Work out the finished part from the listing and answer in its coordinate system (mm). Face numbers are marked on the shaded views. A direction names the side the tool comes from. Round coordinates to 2 decimals unless told otherwise and drop trailing zeros. Loops run counter-clockwise (first coordinate to the right, second up) from the corner with the lowest first, then second, coordinate; pieces in that order, holes last. Notation, with made-up numbers: (23.25, 18) - (45.25, 18) arc R5 ccw to (45.25, 23) - close; hole circle Ø4 at (-21, -1). An arc over 180 degrees is marked (long way). Return JSON: item names as keys, results as strings.
from build123d import *

# Parameters (mm, degrees)
SKETCH1_R           = 2
SKETCH1_R_2         = 13.2
SKETCH1_R_3         = 11.2
BOSS_EXTRUDE1_DEPTH = 3.6
SKETCH2_R           = 2
SKETCH2_R_2         = 5.25
BOSS_EXTRUDE2_DEPTH = 2
SKETCH3_R           = 2
CUT_EXTRUDE1_DEPTH  = 2
SKETCH4_R           = 1.8
BOSS_EXTRUDE3_DEPTH = 3.6


with BuildPart() as part:
    # Sketch1 → Boss-Extrude1 (new body)
    # profile 1 of 3: a face of its own
    with BuildSketch(Plane(origin=(0, 0, 0), x_dir=(1, 0, 0), z_dir=(0, 1, 0))):
        with BuildLine():
            ThreePointArc((-6.939428571, -11.228727938), (-13.2, 0), (-6.939428571, 11.228727938))
            Line((-6.939428571, 11.228727938), (-19.602857143, 3.40264483))
            ThreePointArc((-19.602857143, 3.40264483), (-21.5, 0), (-19.602857143, -3.40264483))
            Line((-19.602857143, -3.40264483), (-6.939428571, -11.228727938))
        make_face()
        with Locations(Location((-17.5, 0, 0), (0, 0, 270))):
            Circle(SKETCH1_R, mode=Mode.SUBTRACT)
    # profile 2 of 3: a face of its own
    with BuildSketch(Plane(origin=(0, 0, 0), x_dir=(1, 0, 0), z_dir=(0, 1, 0))):
        Circle(SKETCH1_R_2)
        with Locations(Location((0, 0, 0), (0, 0, 270))):
            Circle(SKETCH1_R_3, mode=Mode.SUBTRACT)
    # profile 3 of 3: a face of its own
    with BuildSketch(Plane(origin=(0, 0, 0), x_dir=(1, 0, 0), z_dir=(0, 1, 0))):
        with BuildLine():
            Line((19.602857143, 3.40264483), (6.939428571, 11.228727938))
            ThreePointArc((6.939428571, 11.228727938), (11.529103546, 6.428045693), (13.2, 0))
            ThreePointArc((13.2, 0), (11.529103546, -6.428045693), (6.939428571, -11.228727938))
            Line((6.939428571, -11.228727938), (19.602857143, -3.40264483))
            ThreePointArc((19.602857143, -3.40264483), (21.5, 0), (19.602857143, 3.40264483))
        make_face()
        with Locations(Location((17.5, 0, 0), (0, 0, 270))):
            Circle(SKETCH1_R, mode=Mode.SUBTRACT)
    extrude(amount=BOSS_EXTRUDE1_DEPTH)

    # Sketch2 → Boss-Extrude2 (add)
    with BuildSketch(Plane(origin=(0, 3.6, 0), x_dir=(1, 0, 0), z_dir=(0, 1, 0))):
        with BuildLine():
            Line((-6.939428571, 11.228727938), (-19.602857143, 3.40264483))
            ThreePointArc((-19.602857143, 3.40264483), (-21.5, 0), (-19.602857143, -3.40264483))
            Line((-19.602857143, -3.40264483), (-6.939428571, -11.228727938))
            ThreePointArc((-6.939428571, -11.228727938), (0, -13.2), (6.939428571, -11.228727938))
            Line((6.939428571, -11.228727938), (19.602857143, -3.40264483))
            ThreePointArc((19.602857143, -3.40264483), (21.5, 0), (19.602857143, 3.40264483))
            Line((19.602857143, 3.40264483), (6.939428571, 11.228727938))
            ThreePointArc((6.939428571, 11.228727938), (0, 13.2), (-6.939428571, 11.228727938))
        make_face()
        with Locations(Location((17.5, 0, 0), (0, 0, 270))):
            Circle(SKETCH2_R, mode=Mode.SUBTRACT)
        with Locations(Location((-17.5, 0, 0), (0, 0, 270))):
            Circle(SKETCH2_R, mode=Mode.SUBTRACT)
        with Locations(Location((0, 0, 0), (0, 0, 270))):
            Circle(SKETCH2_R_2, mode=Mode.SUBTRACT)
    extrude(amount=BOSS_EXTRUDE2_DEPTH)

    # Sketch3 → Cut-Extrude1 (cut)
    with BuildSketch(Plane(origin=(0, 5.6, 0), x_dir=(1, 0, 0), z_dir=(0, 1, 0))):
        with Locations(Location((5.727564928, 5.727564928, 0), (0, 0, 270))):
            Circle(SKETCH3_R)
        with Locations(Location((-5.727564928, -5.727564928, 0), (0, 0, 270))):
            Circle(SKETCH3_R)
    extrude(amount=-CUT_EXTRUDE1_DEPTH, mode=Mode.SUBTRACT)

    # Sketch4 → Boss-Extrude3 (add)
    with BuildSketch(Plane.XZ.offset(-3.6)):
        with Locations(Location((5.727564928, 5.727564928, 0), (0, 0, 90))):
            Circle(SKETCH4_R)
        with Locations(Location((-5.727564928, -5.727564928, 0), (0, 0, 90))):
            Circle(SKETCH4_R)
    extrude(amount=BOSS_EXTRUDE3_DEPTH)


solid = part.part
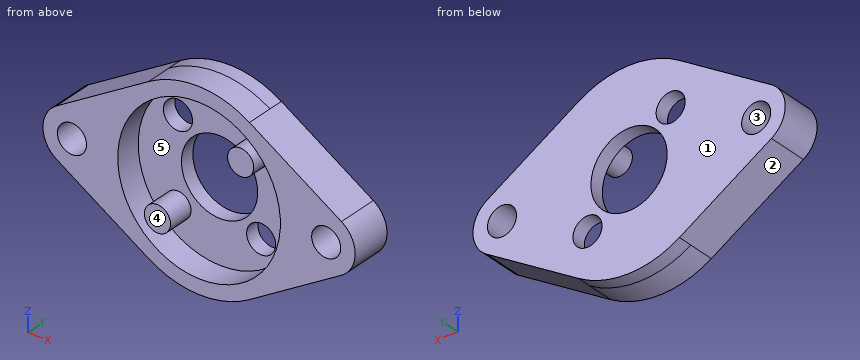
1) Determine the mould class of the marked faces 1, 2 and 3 for opening direction X: pulls with the +X half, pulls with the -X half, needs draft (parallel to the pull), parting line crosses it, or undercut.
Verdict:
{"face 1": "needs draft", "face 2": "pulls with the -X half", "face 3": "undercut"}
2) Flat-ended cylindrical pins translate along their axes: pin 1 (3 mm diameter, centred on x = 0, z = -9, fed in from -Y); pin 2 (2 mm diameter, centred on x = 6, y = 4.5, fed in from +Z); pin 3 (2 mm diameter, centred on x = 12.5, y = 1.5, fed in from -Z). Find the tip coordinate at first contact, or state that the pin passes through.
Verdict:
{"pin 1": "stops at y = 3.6", "pin 2": "stops at z = 12.22", "pin 3": "stops at z = -8.41"}
3) Section C-C (x = 17.5) is taken. Give the vertices of the cut face in (y, z).
Verdict:
{"outline": "(0, -4.7) - (5.6, -4.7) - (5.6, -2) - (0, -2) - close; (0, 2) - (5.6, 2) - (5.6, 4.7) - (0, 4.7) - close"}
4) Section A-A (z = 0) is taken. Give the vertices of the cut face in (x, y), and give its area (3 significant figures).
Verdict:
{"outline": "(-21.5, 0) - (-19.5, 0) - (-19.5, 5.6) - (-21.5, 5.6) - close; (-15.5, 0) - (-11.2, 0) - (-11.2, 3.6) - (-5.25, 3.6) - (-5.25, 5.6) - (-15.5, 5.6) - close; (5.25, 3.6) - (11.2, 3.6) - (11.2, 0) - (15.5, 0) - (15.5, 5.6) - (5.25, 5.6) - close; (19.5, 0) - (21.5, 0) - (21.5, 5.6) - (19.5, 5.6) - close", "area": "94.4 mm2"}
5) Find the intervals of material crossed by L1, parallel to X at y = 0.85, z = 6.75; L2, parallel to X at y = 1.5, z = -0.5; L3, parallel to X at y = 3.15, z = 6.5, in increasing order.
Verdict:
{"L1": "x = -14.19 to -8.94, 4.25 to 7.21, 8.94 to 14.19", "L2": "x = -21.47 to -19.44, -15.56 to -11.19, 11.19 to 15.56, 19.44 to 21.47", "L3": "x = -14.59 to -9.12, 4.1 to 7.35, 9.12 to 14.59"}
6) Section D-D (z = 9.5) is taken. Give the vertices of the cut face in (x, y).
Verdict:
{"outline": "(-9.74, 0) - (-5.93, 0) - (-5.93, 3.6) - (5.93, 3.6) - (5.93, 0) - (9.74, 0) - (9.74, 5.6) - (-9.74, 5.6) - close"}
7) A tool of negligible diameter and unlimited length cuts with its end or side. For the marked faces 4 and 5, from which of +Z, -Z, +X, -X, +Y, -Y can it reach the whole face along a straight path? Write none if from no direction.
Verdict:
{"face 4": "+Z, -Z, +X, -X, -Y", "face 5": "-Y"}
8) Section B-B (y = 1.95) is taken. Give the vertices of the cut face in (x, z), and give its area (3 significant figures).
Verdict:
{"outline": "(-19.6, -3.4) - (-6.94, -11.23) arc R13.2 ccw to (6.94, -11.23) - (19.6, -3.4) arc R4 ccw to (19.6, 3.4) - (6.94, 11.23) arc R13.2 ccw to (-6.94, 11.23) - (-19.6, 3.4) arc R4 ccw to start; circle Ø3.6 at (-5.73, -5.73); circle Ø3.6 at (5.73, 5.73); hole circle Ø4 at (-17.5, 0); hole circle Ø22.4 at (0, 0); hole circle Ø4 at (17.5, 0)", "area": "339 mm2"}
